from build123d import *

# Parameters (mm, degrees)
SKETCH1_W           = 20
SKETCH1_H           = 70
BOSS_EXTRUDE1_DEPTH = 10
SKETCH2_W           = 20
SKETCH2_H           = 10
BOSS_EXTRUDE2_DEPTH = 50
SKETCH3_W           = 20
SKETCH3_H           = 10
BOSS_EXTRUDE3_DEPTH = 7
SKETCH4_W           = 15
SKETCH4_H           = 7
SKETCH4_W_2         = 20
BOSS_EXTRUDE4_DEPTH = 30
SKETCH5_R           = 4.414464055
BOSS_EXTRUDE5_DEPTH = 3


with BuildPart() as part:
    # Sketch1 → Boss-Extrude1 (new body)
    with BuildSketch(Plane.XY):
        with Locations((10, 35)):
            Rectangle(SKETCH1_W, SKETCH1_H)
    extrude(amount=BOSS_EXTRUDE1_DEPTH)

    # Sketch2 → Boss-Extrude2 (add)
    with BuildSketch(Plane.XY.offset(10)):
        with Locations((10, 5)):
            Rectangle(SKETCH2_W, SKETCH2_H)
    extrude(amount=BOSS_EXTRUDE2_DEPTH)

    # Sketch3 → Boss-Extrude3 (add)
    with BuildSketch(Plane.XY.offset(60)):
        with Locations((10, 5)):
            Rectangle(SKETCH3_W, SKETCH3_H)
    extrude(amount=BOSS_EXTRUDE3_DEPTH)

    # Sketch4 → Boss-Extrude4 (add)
    with BuildSketch(Plane(origin=(0, 10, 0), x_dir=(1, 0, 0), z_dir=(0, 1, 0))):
        with Locations((-7.5, -63.5)):
            Rectangle(SKETCH4_W, SKETCH4_H)
        with Locations((10, -63.5)):
            Rectangle(SKETCH4_W_2, SKETCH4_H)
        with Locations((27.5, -63.5)):
            Rectangle(SKETCH4_W, SKETCH4_H)
    extrude(amount=BOSS_EXTRUDE4_DEPTH)

    # Sketch5 → Boss-Extrude5 (add)
    with BuildSketch(Plane.XY.offset(67)):
        with Locations((9.957681606, 29.754854133)):
            Circle(SKETCH5_R)
    extrude(amount=BOSS_EXTRUDE5_DEPTH)


solid = part.part
Input: part model. Units: mm. Frame: model coordinates. A direction names the side the tool comes from. Give positions to 0.01 mm unless a question says otherwise; leave off trailing zeros. Write each loop counter-clockwise with the first axis right and the second up, starting at its lowest first coordinate (ties: lowest second). Pieces come first, ordered by that corner, then holes. Notation, with made-up numbers: M 84.5,-31.5 L 102.5,-31.5 A11 ccw 102.5,-11.5 Z; hole C 24,55.25 d9. An arc over 180 degrees is marked long. Write item = value, one per line. Start each with the question number.
1) First-contact query: pin 1 Ø1.5 at (y, z) = (9.5, 35.5) entering from +X; pin 2 Ø20 at (y, z) = (51, 44.5) entering from -X; pin 3 Ø7.5 at (x, z) = (-10.5, 64) entering from -Y; pin 4 Ø12 at (x, z) = (23.5, 57.5) entering from +Y. Flat tips, straight axial feed; report the tip coordinate or a pass-through.
2) Cut plane C-C on z = 30. Return the cut outline in (x, y), then the cut area to 3 significant figures.
3) Material intervals for line 1 along Z through (x, y) = (9, 21.5); line 2 along Y through (x, z) = (1, 37); line 3 along Z through (x, y) = (-2, 28), sorted ascending. Write a range as [from, to].
4) Cut plane A-A on y = 15. Return the cut outline in (x, z).
5) Draft query along Z for faces 5 (the cylindrical face through (9.38, 34.13, 68.48)), 6 (the flat face through (10, 35, 0)), 7 (the flat face through (10, 40, 10)), 8 (the flat face through (10, 10, 35)). Return one class per face: +Z half, -Z half, draft (parallel to the pull), parting line (faces both ways), or undercut.
6) Cut plane B-B on x = 4. Return the cut outline in (y, z), then the cut area to 3 significant figures.
7) Reachability of faces 1 (the flat face through (27, 10, 63)), 2 (the flat face through (-8, 10, 63)), 3 (the flat face through (10, 25, 60)), 4 (the flat face through (10, 40, 63)) from +Z, -Z, +X, -X, +Y, -Y: full face, straight path, thin tool, end or side. Return the list, or none.
Solved:
q1.pin_1 = 20
q1.pin_2 = through
q1.pin_3 = 10
q1.pin_4 = 40
q2.outline = M 0,0 L 20,0 L 20,10 L 0,10 Z
q2.area = 200 mm2
q3.line_1 = [0, 10], [60, 67]
q3.line_2 = [0, 10]
q3.line_3 = [60, 67]
q4.outline = M -15,60 L 35,60 L 35,67 L -15,67 Z; M 0,0 L 20,0 L 20,10 L 0,10 Z
q5.face_5 = draft
q5.face_6 = -Z half
q5.face_7 = undercut
q5.face_8 = undercut
q6.outline = M 0,0 L 70,0 L 70,10 L 10,10 L 10,60 L 40,60 L 40,67 L 0,67 Z
q6.area = 1,480 mm2
q7.face_1 = +Z, -Z, +X, -Y
q7.face_2 = +Z, -Z, -X, -Y
q7.face_3 = +X, -X, +Y
q7.face_4 = +Z, +X, -X, +Y
